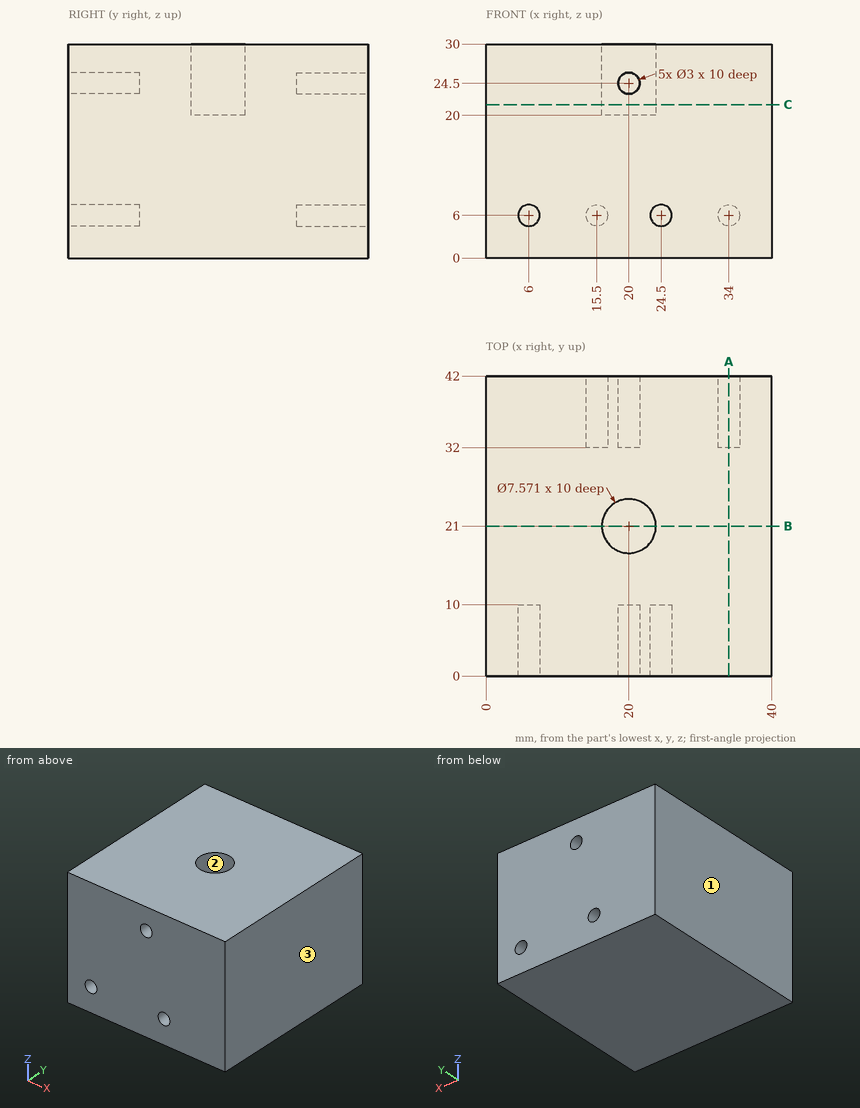
Study the drawing (mm; zero at the part's minimum x, y, z) and answer. Round coordinates to 2 decimals unless told otherwise and drop trailing zeros. Write each loop counter-clockwise with the first axis right and the second up, starting at its lowest first coordinate (ties: lowest second). Pieces come first, ordered by that corner, then holes. Notation, with made-up numbers: (-22.75, -40) - (-8.75, -40) arc R29 ccw to (-8.75, -14) - close; hole circle Ø6 at (0, -28.75). An arc over 180 degrees is marked (long way). Use a Markdown table: item, result. Add a question column.
1. Flat-ended cylindrical pins translate along their axes: P1, Ø0.9, axis at x = 20.5, z = 25, coming from the +Y side; P2, Ø2.5, axis at x = 6, z = 6, coming from the -Y side. Find the tip coordinate at first contact, or state that the pin passes through.
2. The part is cut by section A-A (x = 34). Write down the section's boundary in (y, z), and give its area (3 significant figures).
3. For a pull along X with two mould halves and no side action, classify the marked faces 1, 2 and 3 as +X half, -X half, draft (parallel to the pull), parting line (faces both ways), or undercut.
4. The part is cut by section C-C (z = 21.5). Write down the section's boundary in (x, y) (1 decimal), and give its area (4 significant figures).
5. Consider line 1 (X direction, y = 36.25, z = 6); line 2 (Z direction, x = 20, y = 8); line 3 (Z direction, x = 34, y = 39.75). Determine where each line is inside the solid, lowest interval first.
6. The part is cut by section B-B (y = 21). Write down the section's boundary in (x, z) (1 decimal).
Reported:
| question | item | result |
|---|---|---|
| 1 | P1 | y = 32 |
| 1 | P2 | y = 10 |
| 2 | outline | (0, 0) - (42, 0) - (42, 4.5) - (32, 4.5) - (32, 7.5) - (42, 7.5) - (42, 30) - (0, 30) - close |
| 2 | area | 1,230 mm^2 |
| 3 | face 1 | -X half |
| 3 | face 2 | undercut |
| 3 | face 3 | +X half |
| 4 | outline | (0, 0) - (40, 0) - (40, 42) - (0, 42) - close; hole circle Ø7.6 at (20, 21) |
| 4 | area | 1,635 mm^2 |
| 5 | line 1 | 0 to 14, 17 to 32.5, 35.5 to 40 |
| 5 | line 2 | 0 to 23, 26 to 30 |
| 5 | line 3 | 0 to 4.5, 7.5 to 30 |
| 6 | outline | (0, 0) - (40, 0) - (40, 30) - (23.8, 30) - (23.8, 20) - (16.2, 20) - (16.2, 30) - (0, 30) - close |
